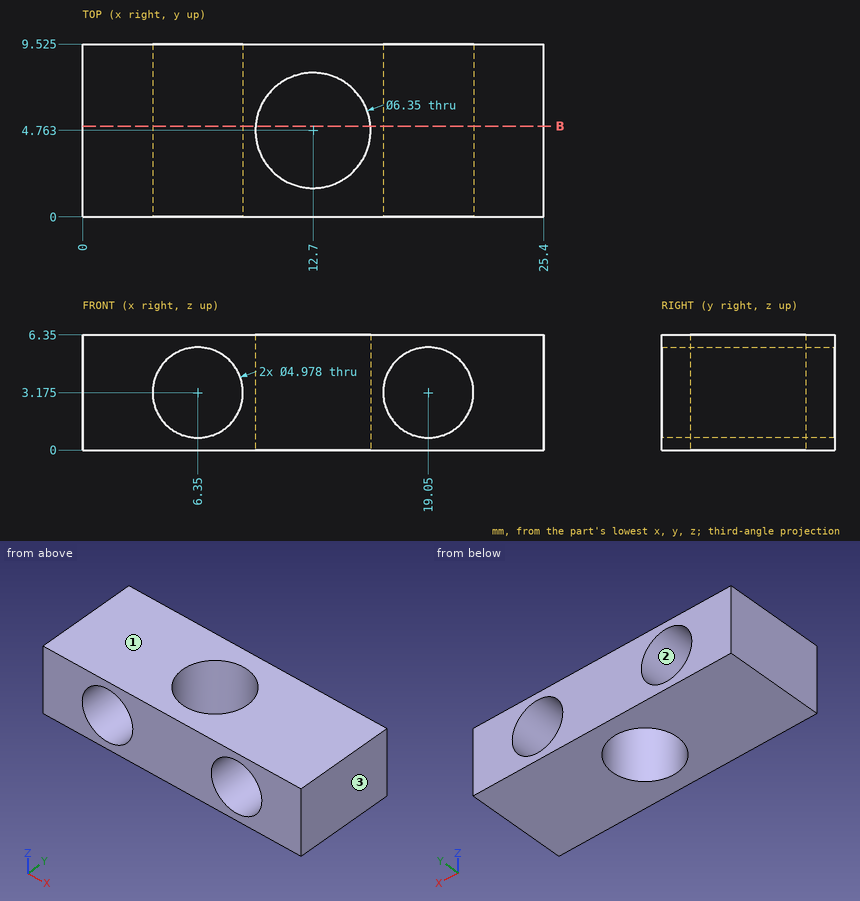
Geometry: see drawing. Coordinates: mm, zero at the bounding-box minimum. Round coordinates to 2 decimals unless told otherwise and drop trailing zeros. Write item = value, one per line. Start each with the question number.
(1) Pull-direction query (Z, two-part tool) for the marked faces 1, 2 and 3; classes: +Z half, -Z half, draft (parallel to the pull), parting line (faces both ways), or undercut.
(2) Ray query, line 1 along X through (y, z) = (8, 3); line 2 along Z through (x, y) = (19, 3); line 3 along X through (y, z) = (8.5, 4.75) (1 decimal). Return the intervals inside material, ascending. Write a range as from..to.
(3) Pin query (flat end, axial travel): pin 1 (4 mm diameter, centred on x = 12.7, y = 4.76, fed in from +Z); pin 2 (1.5 mm diameter, centred on x = 10, y = 3.5, fed in from +Z). Return the tip coordinate at first contact, or that it passes through.
(4) Section query B-B, the plane y = 5. State how many separate pieces and enclosed holes the cut face has.
Conclusion:
q1.face_1 = +Z half
q1.face_2 = undercut
q1.face_3 = draft
q2.line_1 = 0..3.87, 8.83..16.57, 21.53..25.4
q2.line_2 = 0..0.69, 5.66..6.35
q2.line_3 = 0..4.4, 8.3..17.1, 21..25.4
q3.pin_1 = through
q3.pin_2 = 6.35
q4.separate_pieces = 2
q4.enclosed_holes = 2
